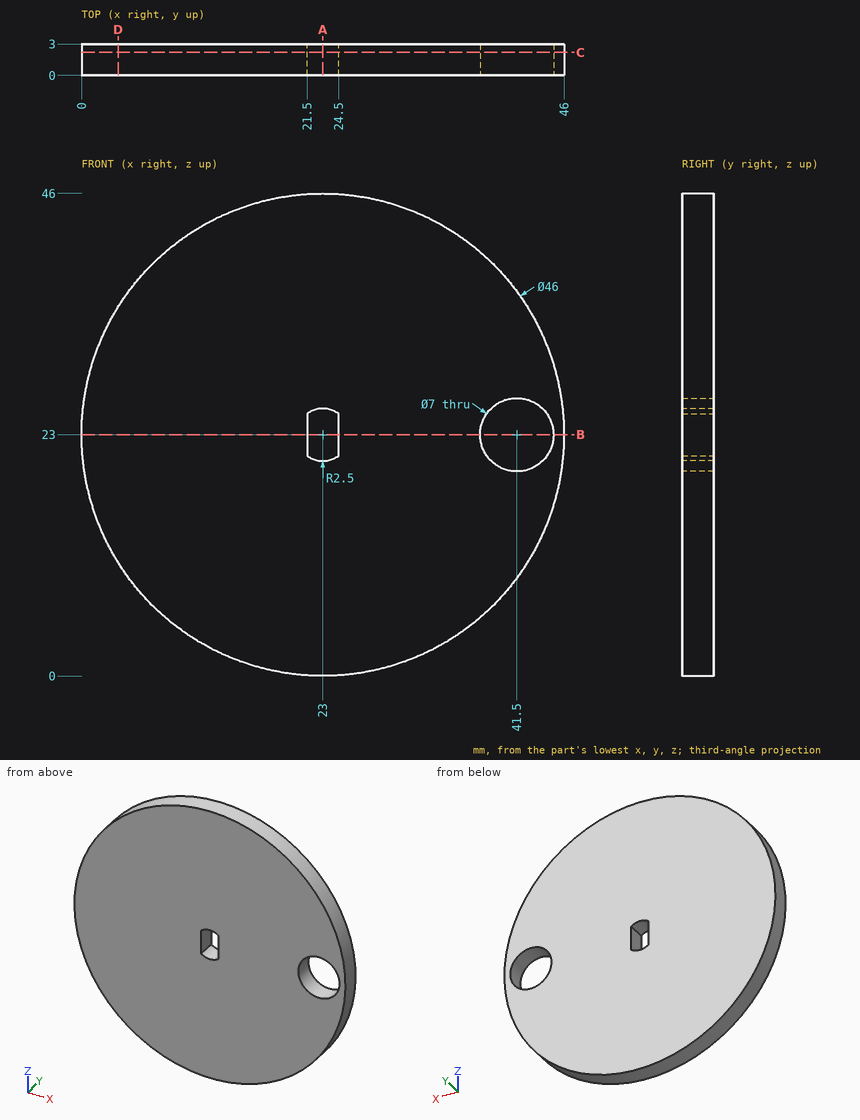
The drawing under review shows one solid part. Ordinate dimensions are in mm from its lowest x, y, z. Round coordinates to 2 decimals unless told otherwise and drop trailing zeros. Write each loop counter-clockwise with the first axis right and the second up, starting at its lowest first coordinate (ties: lowest second). Pieces come first, ordered by that corner, then holes. Notation, with made-up numbers: (-35, 60.5) - (-11, 60.5) arc R35 ccw to (-11, 92.5) - close; hole circle Ø9 at (2.25, -34). An arc over 180 degrees is marked (long way). One line per question, with ' | ' between items.
Item 1: Add section D-D, the plane x = 3.5. Give the boundary of the cut face in (y, z).
Resolved:
outline: (0, 10.8) - (3, 10.8) - (3, 35.2) - (0, 35.2) - close
Item 2: Add section C-C, the plane y = 2.2. Give the boundary of the cut face in (x, z).
Resolved:
outline: circle Ø46 at (23, 23); hole (21.5, 21) arc R2.5 ccw to (24.5, 21) - (24.5, 25) arc R2.5 ccw to (21.5, 25) - close; hole circle Ø7 at (41.5, 23)
Item 3: Add section B-B, the plane z = 23. Give the boundary of the cut face in (x, y).
Resolved:
outline: (0, 0) - (21.5, 0) - (21.5, 3) - (0, 3) - close; (24.5, 0) - (38, 0) - (38, 3) - (24.5, 3) - close; (45, 0) - (46, 0) - (46, 3) - (45, 3) - close
Item 4: To check wall thickness, follow probe 1 along Z at (x, y) = (22, 2.35); probe 2 along Z at (x, y) = (4, 0.35); probe 3 along X at (y, z) = (2.8, 36). State the ranges of each line that lie inside material, in increasing order.
Resolved:
probe 1: z = 0.02 to 20.71, 25.29 to 45.98 | probe 2: z = 10.04 to 35.96 | probe 3: x = 4.03 to 41.97
Item 5: Add section A-A, the plane x = 23. Give the boundary of the cut face in (y, z).
Resolved:
outline: (0, 0) - (3, 0) - (3, 20.5) - (0, 20.5) - close; (0, 25.5) - (3, 25.5) - (3, 46) - (0, 46) - close
Item 6: For P1, Ø1.5, axis at x = 35.5, y = 1, coming from the +Z side; P2, Ø0.9, axis at y = 2, z = 23, coming from the +X side, all flat-tipped, find the tip position at first contact; note any pin that passes through.
Resolved:
P1: stops at z = 42.77 | P2: stops at x = 46
